Verification items for the finished model (mm, model axes). A direction names the side the tool comes from. Coordinates: 2 decimals unless noted, no trailing zeros. Write each loop counter-clockwise with the first axis right and the second up, starting at its lowest first coordinate (ties: lowest second). Pieces come first, ordered by that corner, then holes. Notation, with made-up numbers: (73.25, -13) - (78.25, -13) arc R20 ccw to (78.25, 13) - close; hole circle Ø2 at (74, -0.5). An arc over 180 degrees is marked (long way). Answer as CSV lines item,"result". Start each with the question number.
```python
from build123d import *

# Parameters (mm, degrees)
SKETCH1_W           = 15
SKETCH1_H           = 80
BOSS_EXTRUDE1_DEPTH = 22
CUT_EXTRUDE1_DEPTH  = 23
CUT_EXTRUDE2_DEPTH  = 6
CHAMFER1_SIZE       = 1
SKETCH6_W           = 4.9
SKETCH6_H           = 0.3
BOSS_EXTRUDE2_DEPTH = 5
FILLET2_R           = 1


with BuildPart() as part:
    # Sketch1 → Boss-Extrude1 (new body)
    with BuildSketch(Plane(origin=(0, 0, 0), x_dir=(0, 0, -1), z_dir=(1, 0, 0))):
        with Locations((-7.5, 40)):
            Rectangle(SKETCH1_W, SKETCH1_H)
    extrude(amount=BOSS_EXTRUDE1_DEPTH)

    # Sketch2 → Cut-Extrude1 (cut, through all)
    with BuildSketch(Plane(origin=(22, 0, 0), x_dir=(0, 0, -1), z_dir=(1, 0, 0))):
        with BuildLine():
            Line((-15, 80), (-15, 13.1))
            Line((-15, 13.1), (-10.1, 13.1))
            Line((-10.1, 13.1), (-10.1, 10.55))
            ThreePointArc((-10.1, 10.55), (-7.55, 8), (-5, 10.55))
            Line((-5, 10.55), (-5, 80))
            Line((-5, 80), (-15, 80))
        make_face()
    extrude(amount=-CUT_EXTRUDE1_DEPTH, mode=Mode.SUBTRACT)

    # Sketch3 → Cut-Extrude2 (cut, through all)
    with BuildSketch(Plane.XY.offset(5)):
        with BuildLine():
            Line((7, 74.1), (15, 74.1))
            ThreePointArc((15, 74.1), (17.1, 72), (15, 69.9))
            Line((15, 69.9), (7, 69.9))
            ThreePointArc((7, 69.9), (4.9, 72), (7, 74.1))
        make_face()
    extrude(amount=-CUT_EXTRUDE2_DEPTH, mode=Mode.SUBTRACT)

    # Chamfer1
    chamfer1_edges = [part.edges().sort_by_distance(p)[0] for p in [
        (4.9, 72, 5),
        (11, 69.9, 5),
        (17.1, 72, 5),
        (11, 74.1, 5),
    ]]
    chamfer(chamfer1_edges, length=CHAMFER1_SIZE)

    # Sketch6 → Boss-Extrude2 (add)
    with BuildSketch(Plane.ZY):
        Polygon((10.1, 13.4), (15, 13.4), (15, 15.4), (5.5, 15.4), (5.5, 13.4), align=None)
        with Locations((12.55, 13.25)):
            Rectangle(SKETCH6_W, SKETCH6_H)
    extrude(amount=-BOSS_EXTRUDE2_DEPTH)

    # Fillet2
    fillet2_edges = [part.edges().sort_by_distance(p)[0] for p in [
        (5, 14.25, 15),
        (11, 0, 0),
        (11, 80, 0),
        (11, 80, 5),
        (13.5, 13.1, 15),
        (11, 0, 15),
        (2.5, 15.4, 15),
        (5, 13.1, 12.55),
    ]]
    fillet(fillet2_edges, radius=FILLET2_R)


solid = part.part
```
1. Depth check by flat-ended pin: P1, Ø12, axis at x = 12, y = 20.5, coming from the +Z side; P2, Ø5.5, axis at x = 2.5, z = 8.5, coming from the +Y side; P3, Ø2, axis at x = 15.5, z = 11, coming from the +Y side; P4, Ø3, axis at y = 60, z = 7.5, coming from the -X side. Enter the tip coordinate at first touch or a pass-through.
2. Draft check along Z on faces 1 (the face through (2, 15.4, 10)), 2 (the face through (11, 8, 15)), 3 (the face through (3, 14, 5.5)), 4 (the face through (3, 13.4, 8)). Enter one of: pulls with the +Z half, pulls with the -Z half, needs draft (parallel to the pull), parting line crosses it, or undercut.
3. Cross-section at D-D (z = 2.5). Record the cut outline in (x, y), and give its area (3 significant figures).
4. Cross-section at A-A (x = 10.25). Record the cut outline in (y, z).
5. Cross-section at B-B (y = 72). Record the cut outline in (x, z), and give its area (3 significant figures).
6. Cross-section at C-C (z = 7.55). Record the cut outline in (x, y), and give its area (3 significant figures).
7. Scan lines: line 1 along Z through (x, y) = (21, 11.5); line 2 along Y through (x, z) = (3.25, 7.75); line 3 along Y through (x, z) = (18.5, 12.25). Record each from-to range of solid material in increasing order. Write a range as from..to.
8. Access from +Z, -Z, +X, -X, +Y, -Y to the whole of each face (thin tool, end or side, straight path). Record for faces 5 (the face through (11, 69.9, 2)), 6 (the face through (4.7, 72, 4.2)), 7 (the face through (5, 15, 10)).
Completed:
1,P1,"stops at z = 5"
1,P2,"stops at y = 15.4"
1,P3,"stops at y = 13.1"
1,P4,"passes through"
2,face 1,"needs draft"
2,face 2,"pulls with the +Z half"
2,face 3,"undercut"
2,face 4,"undercut"
3,outline,"(0, 0) - (22, 0) - (22, 80) - (0, 80) - close; hole (7, 69.9) - (15, 69.9) arc R2.1 ccw to (15, 74.1) - (7, 74.1) arc R2.1 ccw to start"
3,area,"1,710 mm2"
4,outline,"(0, 1) arc R1 ccw to (1, 0) - (69.9, 0) - (69.9, 4) - (68.9, 5) - (10.55, 5) arc R2.55 cw to (10.55, 10.1) - (13.1, 10.1) - (13.1, 14) arc R1 ccw to (12.1, 15) - (1, 15) arc R1 ccw to (0, 14) - close; (74.1, 0) - (79, 0) arc R1 ccw to (80, 1) - (80, 4) arc R1 ccw to (79, 5) - (75.1, 5) - (74.1, 4) - close"
5,outline,"(0, 0) - (4.9, 0) - (4.9, 4) - (3.9, 5) - (0, 5) - close; (17.1, 0) - (22, 0) - (22, 5) - (18.1, 5) - (17.1, 4) - close"
5,area,"48.0 mm2"
6,outline,"(0, 0) - (22, 0) - (22, 8) - (0, 8) - close; (0, 13.4) - (5.29, 13.4) arc R1 cw to (5, 14.1) - (5, 15.4) - (0, 15.4) - close"
6,area,"186 mm2"
7,line 1,"z = 0..5, 10.1..15"
7,line 2,"y = 0..8.01, 13.4..15.4"
7,line 3,"y = 0..13.1"
8,face 5,"+Z, -Z"
8,face 6,"+Z"
8,face 7,"+Z, +X, +Y"
